from build123d import *

# Parameters (mm, degrees)
MASS_DEPTH          = 6.35
SKETCH4_R           = 3.175
CUT_EXTRUDE1_DEPTH  = 127.253666407
SKETCH3_W           = 12.7
SKETCH3_H           = 12.7
CUT_EXTRUDE2_DEPTH  = 127.253666407
LPATTERN1_COUNT     = 7
LPATTERN1_PITCH     = 25.4
SKETCH5_R           = 7.9375
CUT_EXTRUDE3_DEPTH  = 127.253666407
LPATTERN2_COUNT     = 4
LPATTERN2_PITCH     = 25.4
CAVITY1_START       = 53.18125
CAVITY1_OUTLINE_W   = 11.1125
CAVITY1_OUTLINE_H   = 6.35
CAVITY1_DEPTH       = 6.35
CAVITY1_START_2     = 82.55
CAVITY1_2_OUTLINE_W = 11.1125
CAVITY1_2_OUTLINE_H = 6.35
CAVITY1_2_DEPTH     = 6.35


# Read off the part's stored shape, not the designer's step: Cavity1
with BuildPart() as part:
    # Sketch1 → Mass (new body)
    with BuildSketch(Plane.XY):
        with BuildLine():
            Line((-88.9, -23.8125), (88.9, -23.8125))
            Line((88.9, -23.8125), (88.9, 23.8125))
            Line((88.9, 23.8125), (-88.9, 23.8125))
            Line((-88.9, 23.8125), (-118.664971781, 8.4659699))
            ThreePointArc((-118.664971781, 8.4659699), (-123.825, 0), (-118.664971781, -8.4659699))
            Line((-118.664971781, -8.4659699), (-88.9, -23.8125))
        make_face()
    extrude(amount=MASS_DEPTH)

    # Sketch4 → Cut-Extrude1 (cut, through all)
    with BuildSketch(Plane(origin=(0, 0, 0), x_dir=(-1, 0, 0), z_dir=(0, 0, -1))):
        with Locations((114.3, 0)):
            Circle(SKETCH4_R)
    extrude(amount=-CUT_EXTRUDE1_DEPTH, mode=Mode.SUBTRACT)

    # Sketch3 → Cut-Extrude2 (cut, through all)
    with BuildSketch(Plane(origin=(0, 0, 0), x_dir=(-1, 0, 0), z_dir=(0, 0, -1))):
        with Locations((-82.55, 23.8125)):
            Rectangle(SKETCH3_W, SKETCH3_H)
        with Locations((-82.55, -23.8125)):
            Rectangle(SKETCH3_W, SKETCH3_H)
    cut_extrude2 = extrude(amount=-CUT_EXTRUDE2_DEPTH, mode=Mode.SUBTRACT)

    # LPattern1: Cut-Extrude2 ×7
    with Locations(*[(-i * LPATTERN1_PITCH, 0, 0) for i in range(1, LPATTERN1_COUNT)]):
        add(cut_extrude2, mode=Mode.SUBTRACT)

    # Sketch5 → Cut-Extrude3 (cut, through all)
    with BuildSketch(Plane.XY.offset(6.35)):
        with Locations((69.85, 0)):
            Circle(SKETCH5_R)
    cut_extrude3 = extrude(amount=-CUT_EXTRUDE3_DEPTH, mode=Mode.SUBTRACT)

    # LPattern2: Cut-Extrude3 ×4
    with Locations(*[(-i * LPATTERN2_PITCH, 0, 0) for i in range(1, LPATTERN2_COUNT)]):
        add(cut_extrude3, mode=Mode.SUBTRACT)

    # Cavity1 outline → Cavity1 (cut)
    with BuildSketch(Plane.YZ.offset(CAVITY1_START)):
        with Locations((-11.90625, 3.175)):
            Rectangle(CAVITY1_OUTLINE_W, CAVITY1_OUTLINE_H)
        with Locations((11.90625, 3.175)):
            Rectangle(CAVITY1_OUTLINE_W, CAVITY1_OUTLINE_H)
    extrude(amount=CAVITY1_DEPTH, mode=Mode.SUBTRACT)

    # Cavity1 2 outline → Cavity1 2 (cut)
    with BuildSketch(Plane.YZ.offset(CAVITY1_START_2)):
        with Locations((-11.90625, 3.175)):
            Rectangle(CAVITY1_2_OUTLINE_W, CAVITY1_2_OUTLINE_H)
        with Locations((11.90625, 3.175)):
            Rectangle(CAVITY1_2_OUTLINE_W, CAVITY1_2_OUTLINE_H)
    extrude(amount=CAVITY1_2_DEPTH, mode=Mode.SUBTRACT)


solid = part.part
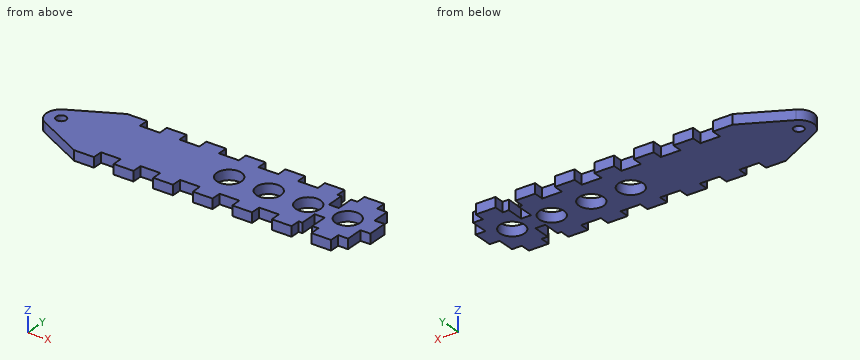
The model under review builds one solid part; all positions refer to its coordinate system, in mm. Give positions to 0.01 mm unless a question says otherwise; leave off trailing zeros. Order: outer loops, then holes, each group sorted by start corner. A loop starts at its lowest first (then second) coordinate and runs counter-clockwise, first axis right, second up. Notation, with made-up numbers: M 60,48 L 75,48 A18 cw 75,80 Z; hole C 21,3 d5. An arc over 180 degrees is marked long. One line per question, with ' | ' between items. Start each with the question number.
1) Consider section C-C, the plane y = -20. Give the boundary of the cut face in (x, z).
2) Consider section A-A, the plane x = 19.05. Give the boundary of the cut face in (y, z).
3) Consider section B-B, the plane y = 0. State how many separate pieces and enclosed holes the cut face has, then the cut area to 3 significant figures.
4) Clearance check with flat-ended pins moving along their axes: P1, Ø1.9, axis at x = 52, z = 1.5, coming from the +Y side; P2, Ø3, axis at y = -21, z = 4, coming from the -X side; P3, Ø0.7, axis at x = 52.5, z = 4.5, coming from the -Y side. State where each tip first meets the part, or that it passes through.
5) Consider section D-D, the plane x = 72. Give the boundary of the cut face in (y, z), then the cut area to 3 significant figures.
6) Wall thickness on L1, parallel to Y at x = -6.35, z = 3.25; L2, parallel to X at y = -2, z = 4.5; L3, parallel to Y at x = 57, z = 5.75: over which ranges is each line inside the solid? List them lowest first. Write a range as from..to.
Found:
1) outline: M -96.29,0 L -76.2,0 L -76.2,6.35 L -96.29,6.35 Z; M -63.5,0 L -50.8,0 L -50.8,6.35 L -63.5,6.35 Z; M -38.1,0 L -25.4,0 L -25.4,6.35 L -38.1,6.35 Z; M -12.7,0 L 0,0 L 0,6.35 L -12.7,6.35 Z; M 12.7,0 L 25.4,0 L 25.4,6.35 L 12.7,6.35 Z; M 38.1,0 L 50.8,0 L 50.8,6.35 L 38.1,6.35 Z; M 63.5,0 L 76.2,0 L 76.2,6.35 L 63.5,6.35 Z
2) outline: M -23.81,0 L -7.94,0 L -7.94,6.35 L -23.81,6.35 Z; M 7.94,0 L 23.81,0 L 23.81,6.35 L 7.94,6.35 Z
3) separate pieces: 6 | enclosed holes: 0 | area: 907 mm²
4) P1: stops at y = 17.46 | P2: stops at x = -97.26 | P3: stops at y = -17.46
5) outline: M -23.81,0 L -7.64,0 L -7.64,6.35 L -23.81,6.35 Z; M 7.64,0 L 23.81,0 L 23.81,6.35 L 7.64,6.35 Z | area: 205 mm²
6) L1: y = -23.81..-7.94, 7.94..23.81 | L2: x = -123.61..-116.77, -111.83..-14.03, 1.33..11.37, 26.73..36.77, 52.13..62.17, 77.53..88.9 | L3: y = -6.35..6.35
